Read the model definition and answer for the solid it produces. Units are mm, in the model's axes. Face numbers are marked on the shaded views. Give positions to 0.01 mm unless a question says otherwise; leave off trailing zeros. Order: outer loops, then holes, each group sorted by start corner. A loop starts at its lowest first (then second) coordinate and runs counter-clockwise, first axis right, second up. Notation, with made-up numbers: (-18, -37.75) - (31, -37.75) arc R13 cw to (31, -18.75) - close; hole circle Ø9 at (-14.5, 27.5). An arc over 180 degrees is marked (long way). Return JSON: item names as keys, results as strings.
```python
from build123d import *

# Parameters (mm, degrees)
ESQUISSE1_W             = 30
ESQUISSE1_H             = 60
BOSS_EXTRU_1_DEPTH      = 5
ENL_V_MAT_EXTRU_1_REACH = 35.912
ESQUISSE2_R             = 3.175
ESQUISSE2_R_2           = 3.25
ESQUISSE2_R_3           = 3.325
ESQUISSE2_R_4           = 3.425
ESQUISSE2_R_5           = 3.5
ESQUISSE2_R_6           = 3.575
ESQUISSE2_R_7           = 3.225
CONG_1_R                = 10


with BuildPart() as part:
    # Esquisse1 → Boss.-Extru.1 (new body)
    with BuildSketch(Plane(origin=(0, 0, 0), x_dir=(1, 0, 0), z_dir=(0, 1, 0))):
        Rectangle(ESQUISSE1_W, ESQUISSE1_H)
    extrude(amount=BOSS_EXTRU_1_DEPTH)

    # Esquisse2 → Enlèv. mat.-Extru.1 (cut, up to next)
    with BuildSketch(Plane(origin=(0, 5, 0), x_dir=(1, 0, 0), z_dir=(0, 1, 0)), mode=Mode.PRIVATE) as enl_v_mat_extru_1_sk1:
        with Locations(Location((0, -20, 0), (0, 0, 270))):
            Circle(ESQUISSE2_R)
    enl_v_mat_extru_1_tool1 = extrude(enl_v_mat_extru_1_sk1.sketch, amount=-ENL_V_MAT_EXTRU_1_REACH, mode=Mode.PRIVATE) & part.part
    # Esquisse2 → Enlèv. mat.-Extru.1 (cut, up to next)
    with BuildSketch(Plane(origin=(0, 5, 0), x_dir=(1, 0, 0), z_dir=(0, 1, 0)), mode=Mode.PRIVATE) as enl_v_mat_extru_1_sk2:
        with Locations(Location((0, -10, 0), (0, 0, 270))):
            Circle(ESQUISSE2_R_2)
    enl_v_mat_extru_1_tool2 = extrude(enl_v_mat_extru_1_sk2.sketch, amount=-ENL_V_MAT_EXTRU_1_REACH, mode=Mode.PRIVATE) & part.part
    # Esquisse2 → Enlèv. mat.-Extru.1 (cut, up to next)
    with BuildSketch(Plane(origin=(0, 5, 0), x_dir=(1, 0, 0), z_dir=(0, 1, 0)), mode=Mode.PRIVATE) as enl_v_mat_extru_1_sk3:
        with Locations(Location((0, 0, 0), (0, 0, 270))):
            Circle(ESQUISSE2_R_3)
    enl_v_mat_extru_1_tool3 = extrude(enl_v_mat_extru_1_sk3.sketch, amount=-ENL_V_MAT_EXTRU_1_REACH, mode=Mode.PRIVATE) & part.part
    # Esquisse2 → Enlèv. mat.-Extru.1 (cut, up to next)
    with BuildSketch(Plane(origin=(0, 5, 0), x_dir=(1, 0, 0), z_dir=(0, 1, 0)), mode=Mode.PRIVATE) as enl_v_mat_extru_1_sk4:
        with Locations(Location((0, 10, 0), (0, 0, 270))):
            Circle(ESQUISSE2_R_4)
    enl_v_mat_extru_1_tool4 = extrude(enl_v_mat_extru_1_sk4.sketch, amount=-ENL_V_MAT_EXTRU_1_REACH, mode=Mode.PRIVATE) & part.part
    # Esquisse2 → Enlèv. mat.-Extru.1 (cut, up to next)
    with BuildSketch(Plane(origin=(0, 5, 0), x_dir=(1, 0, 0), z_dir=(0, 1, 0)), mode=Mode.PRIVATE) as enl_v_mat_extru_1_sk5:
        with Locations(Location((0, 20, 0), (0, 0, 270))):
            Circle(ESQUISSE2_R_5)
    enl_v_mat_extru_1_tool5 = extrude(enl_v_mat_extru_1_sk5.sketch, amount=-ENL_V_MAT_EXTRU_1_REACH, mode=Mode.PRIVATE) & part.part
    # Esquisse2 → Enlèv. mat.-Extru.1 (cut, up to next)
    with BuildSketch(Plane(origin=(0, 5, 0), x_dir=(1, 0, 0), z_dir=(0, 1, 0)), mode=Mode.PRIVATE) as enl_v_mat_extru_1_sk6:
        with Locations(Location((8, -15, 0), (0, 0, 270))):
            Circle(ESQUISSE2_R_6)
    enl_v_mat_extru_1_tool6 = extrude(enl_v_mat_extru_1_sk6.sketch, amount=-ENL_V_MAT_EXTRU_1_REACH, mode=Mode.PRIVATE) & part.part
    # Esquisse2 → Enlèv. mat.-Extru.1 (cut, up to next)
    with BuildSketch(Plane(origin=(0, 5, 0), x_dir=(1, 0, 0), z_dir=(0, 1, 0)), mode=Mode.PRIVATE) as enl_v_mat_extru_1_sk7:
        with Locations(Location((-7.5, 15, 0), (0, 0, 270))):
            Circle(ESQUISSE2_R_7)
    enl_v_mat_extru_1_tool7 = extrude(enl_v_mat_extru_1_sk7.sketch, amount=-ENL_V_MAT_EXTRU_1_REACH, mode=Mode.PRIVATE) & part.part
    add(enl_v_mat_extru_1_tool1.solids().sort_by_distance((0, 5, 20))[0], mode=Mode.SUBTRACT)
    add(enl_v_mat_extru_1_tool2.solids().sort_by_distance((0, 5, 10))[0], mode=Mode.SUBTRACT)
    add(enl_v_mat_extru_1_tool3.solids().sort_by_distance((0, 5, 0))[0], mode=Mode.SUBTRACT)
    add(enl_v_mat_extru_1_tool4.solids().sort_by_distance((0, 5, -10))[0], mode=Mode.SUBTRACT)
    add(enl_v_mat_extru_1_tool5.solids().sort_by_distance((0, 5, -20))[0], mode=Mode.SUBTRACT)
    add(enl_v_mat_extru_1_tool6.solids().sort_by_distance((8, 5, 15))[0], mode=Mode.SUBTRACT)
    add(enl_v_mat_extru_1_tool7.solids().sort_by_distance((-7.5, 5, -15))[0], mode=Mode.SUBTRACT)

    # Congé1
    cong_1_edges = [part.edges().sort_by_distance(p)[0] for p in [
        (15, 2.5, -30),
    ]]
    fillet(cong_1_edges, radius=CONG_1_R)


solid = part.part
```
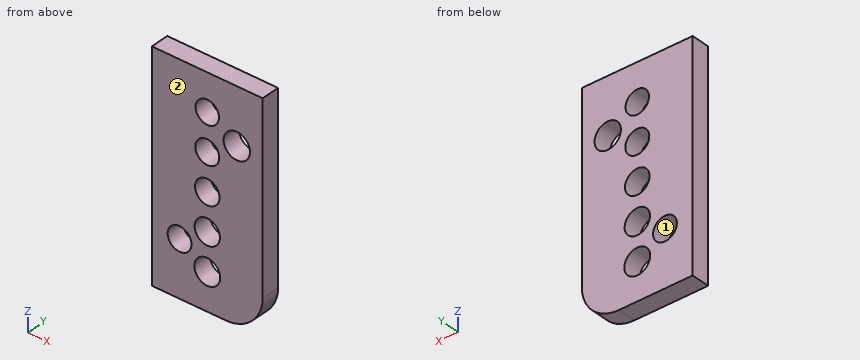
Q1. A cutting plane is placed at B-B (x = 0). Write down the section's boundary in (y, z) (3 decimals), and give its area (3 significant figures).
Values:
{"outline": "(0, -30) - (5, -30) - (5, -23.5) - (0, -23.5) - close; (0, -16.5) - (5, -16.5) - (5, -13.425) - (0, -13.425) - close; (0, -6.575) - (5, -6.575) - (5, -3.325) - (0, -3.325) - close; (0, 3.325) - (5, 3.325) - (5, 6.75) - (0, 6.75) - close; (0, 13.25) - (5, 13.25) - (5, 16.825) - (0, 16.825) - close; (0, 23.175) - (5, 23.175) - (5, 30) - (0, 30) - close", "area": "133 mm²"}
Q2. A cutting plane is placed at A-A (z = 0). Write down the section's boundary in (x, y) (3 decimals), and give its area (3 significant figures).
Values:
{"outline": "(-15, 0) - (-3.325, 0) - (-3.325, 5) - (-15, 5) - close; (3.325, 0) - (15, 0) - (15, 5) - (3.325, 5) - close", "area": "117 mm²"}
Q3. Consider L1, parallel to X at y = 3.75, z = 10; L2, parallel to Z at x = 2.5, y = 2; L3, parallel to X at y = 4, z = -15 (3 decimals). Determine where each line is inside the solid, lowest interval first.
Values:
{"L1": "x = -15 to -3.25, 3.25 to 15", "L2": "z = -30 to -22.45, -17.55 to -12.34, -7.66 to -2.19, 2.19 to 7.92, 12.08 to 18.04, 21.96 to 30", "L3": "x = -15 to -10.725, -4.275 to 15"}
Q4. Given pin 1 (6.5 mm diameter, centred on x = 8, z = 15, fed in from +Y), flat-ended and moving along its own axis, determine where the tip first touches the part or whether it passes through.
Values:
{"pin 1": "passes through"}
Q5. A cutting plane is placed at C-C (y = 4.2). Write down the section's boundary in (x, z) (3 decimals).
Values:
{"outline": "(-15, -30) - (5, -30) arc R10 ccw to (15, -20) - (15, 30) - (-15, 30) - close; hole circle Ø6.45 at (-7.5, -15); hole circle Ø7 at (0, -20); hole circle Ø6.85 at (0, -10); hole circle Ø6.65 at (0, 0); hole circle Ø6.5 at (0, 10); hole circle Ø6.35 at (0, 20); hole circle Ø7.15 at (8, 15)"}
Q6. Determine the mould class of the marked faces 1 and 2 for opening direction Z: released by +Z, released by -Z, zero draft, split by the parting line, or undercut.
Values:
{"face 1": "undercut", "face 2": "zero draft"}
Q7. A cutting plane is placed at D-D (x = -7.5). Write down the section's boundary in (y, z) (3 decimals).
Values:
{"outline": "(0, -30) - (5, -30) - (5, -18.225) - (0, -18.225) - close; (0, -11.775) - (5, -11.775) - (5, 30) - (0, 30) - close"}
